The listing builds one solid part. Answer for the finished solid, in the listing's coordinates (mm). Round coordinates to 2 decimals unless told otherwise and drop trailing zeros. Write each loop counter-clockwise with the first axis right and the second up, starting at its lowest first coordinate (ties: lowest second). Pieces come first, ordered by that corner, then holes.
Item 1: Each of these flat-tipped pins is pushed along its axis until it touches: pin 1 (4 mm diameter, centred on x = 9.5, z = 48, fed in from +Y); pin 2 (10 mm diameter, centred on x = 294, z = 124, fed in from -Y). Where does it stop, or does it pass through?
Item 2: Find section C-C on z = 99.5. Give the vertices of the cut face in (x, y), then the cut area to 3 significant figures.
Item 3: Find section D-D on x = 140.5. Give the vertices of the cut face in (y, z), then the cut area to 3 significant figures.
Item 4: For a pull along Y with two mould halves and no side action, classify faces 1 (the face through (144, -276, 0)), 2 (the face through (211.06, -242.37, 72.47)), 3 (the face through (273.398, -546.788, 72.471)) as +Y half, -Y half, draft (parallel to the pull), parting line (faces both ways), or undercut.
Item 5: Find section A-A on x = 14.5. Give the vertices of the cut face in (y, z).
Item 6: Find section B-B on y = -578.5. Give the vertices of the cut face in (x, z), then the cut area to 3 significant figures.
Item 7: Find the intervals of material crossed by probe 1 along X at (y, z) = (-10, 21); probe 2 along Y at (x, z) = (0, 53); probe 3 along Y at (x, z) = (-12.5, 28), in increasing order.
Autodesk Inventor part; units mm, degrees
ref_plane "YZ Plane" through (0, 0, 0) normal (1, 0, 0) x (0, 1, 0)
ref_plane "XZ Plane" through (0, 0, 0) normal (0, 1, 0) x (-1, 0, 0)
ref_plane "XY Plane" through (0, 0, 0) normal (0, 0, 1) x (1, 0, 0)
sketch "Sketch1" plane through (0, 0, 0) normal (0, 0, 1) x (1, 0, 0)
  arc A0 (66.4929, 34.6943) -> (-66.4929, -34.6943) centre (0, 0) ccw
  circle A1 centre (0, 0) radius 25
  arc A2 (226.7447, -596.6943) -> (359.7304, -527.3057) centre (293.2376, -562) ccw
  circle A3 centre (293.2376, -562) radius 25
  line L0 (-66.4929, -34.6943) -> (226.7447, -596.6943)
  line L1 (66.4929, 34.6943) -> (359.7304, -527.3057)
  dimension "d0" = 150
  dimension "d1" = 50
  dimension "d2" = 150
  dimension "d3" = 50
  dimension "d4" = 562
extrude "Extrusion1" add sketch "Sketch1" along normal blind 147
properties part number "FIRST ARM"
Check values:
1. pin 1: stops at y = 74.62
1. pin 2: stops at y = -637
2. outline: (-66.49, -34.69) - (226.74, -596.69) arc R75 ccw to (359.73, -527.31) - (66.49, 34.69) arc R75 ccw to start; hole circle Ø50 at (0, 0); hole circle Ø50 at (293.24, -562)
2. area: 109,000 mm2
3. outline: (-431.4, 0) - (-107.14, 0) - (-107.14, 147) - (-431.4, 147) - close
3. area: 47,700 mm2
4. face 1: draft
4. face 2: +Y half
4. face 3: undercut
5. outline: (-189.92, 0) - (-20.37, 0) - (-20.37, 147) - (-189.92, 147) - close; (20.37, 0) - (73.58, 0) - (73.58, 147) - (20.37, 147) - close
6. outline: (217.25, 0) - (274.46, 0) - (274.46, 147) - (217.25, 147) - close; (312.02, 0) - (366.4, 0) - (366.4, 147) - (312.02, 147) - close
6. area: 16,400 mm2
7. probe 1: x = -74.33 to -22.91, 22.91 to 89.81
7. probe 2: y = -162.13 to -25, 25 to 75
7. probe 3: y = -138.17 to -21.65, 21.65 to 73.95
